```python
from build123d import *

# Parameters (mm, degrees)
SKETCH040_W  = 133
SKETCH040_H  = 133
PAD038_DEPTH = 66.5
PAD039_DEPTH = 5
SKETCH043_W  = 80
SKETCH043_H  = 60
PAD040_DEPTH = 90
PAD046_DEPTH = 5
SKETCH050_W  = 80
SKETCH050_H  = 60
PAD047_DEPTH = 80


with BuildPart() as part:
    # Sketch040 → Pad038 (new body, symmetric)
    with BuildSketch(Plane.XY):
        Rectangle(SKETCH040_W, SKETCH040_H)
    extrude(amount=PAD038_DEPTH, both=True)

    # Sketch041 (on Face6 of Pad038) → Pad039 (join)
    with BuildSketch(Plane.XY.offset(66.5)):
        with BuildLine():
            Line((-88.5, 88.5), (-66.5, 88.5))
            Line((-66.5, 88.5), (-66.5, 67.5))
            ThreePointArc((-67.5, 66.5), (-65.792893, 65.792893), (-66.5, 67.5))
            Line((-88.5, 66.5), (-67.5, 66.5))
            Line((-88.5, 66.5), (-88.5, 88.5))
        make_face()
    extrude(amount=PAD039_DEPTH)

    # Sketch043 (on Face13 of Pad039) → Pad040 (join)
    with BuildSketch(Plane.XY.offset(71.5)):
        with Locations((-77.5, 82.5)):
            Rectangle(SKETCH043_W, SKETCH043_H)
    extrude(amount=PAD040_DEPTH)

    # Sketch049 (on Face13 of Pad040) → Pad046 (join)
    with BuildSketch(Plane.XY.offset(66.5)):
        with BuildLine():
            Line((91, -66.5), (91, -91))
            Line((91, -91), (66.5, -91))
            Line((66.5, -69), (66.5, -91))
            ThreePointArc((69, -66.5), (64.732233, -64.732233), (66.5, -69))
            Line((69, -66.5), (91, -66.5))
        make_face()
    extrude(amount=PAD046_DEPTH)

    # Sketch050 (on Face23 of Pad046) → Pad047 (join)
    with BuildSketch(Plane.XY.offset(71.5)):
        with Locations((78.75, -73.75)):
            Rectangle(SKETCH050_W, SKETCH050_H)
    extrude(amount=PAD047_DEPTH)


solid = part.part
```
The listing builds one solid part. Answer for the finished solid, in the listing's coordinates (mm). A direction names the side the tool comes from. Coordinates: 2 decimals unless noted, no trailing zeros. Write each loop counter-clockwise with the first axis right and the second up, starting at its lowest first coordinate (ties: lowest second). Pieces come first, ordered by that corner, then holes. Notation, with made-up numbers: (75, -25.75) - (116, -25.75) arc R30 ccw to (116, 1.25) - close; hole circle Ø5 at (37, 34). An arc over 180 degrees is marked (long way). One line per item, written item: value.
1) Consider line 1 along Y through (x, z) = (3, -29); line 2 along Z through (x, y) = (41, -83.5). Determine where each line is inside the solid, lowest interval first. Write a range as from..to.
Geometry check:
line 1: y = -66.5..66.5
line 2: z = 71.5..151.5
2) Find section A-A (x = 48). Give the vertices of the cut face in (y, z).
Geometry check:
outline: (-103.75, 71.5) - (-43.75, 71.5) - (-43.75, 151.5) - (-103.75, 151.5) - close; (-66.5, -66.5) - (66.5, -66.5) - (66.5, 66.5) - (-66.5, 66.5) - close
3) Each of these flat-tipped pins is pushed along its axis until it touches: pin 1 Ø4 at (x, z) = (-75, 69) entering from -Y; pin 2 Ø5 at (x, z) = (71, 89) entering from +Y; pin 3 Ø1.5 at (y, z) = (-82, 68) entering from +X; pin 4 Ø12 at (x, z) = (-76, 71) entering from +Y. Where does it stop, or does it pass through?
Geometry check:
pin 1: stops at y = 66.5
pin 2: stops at y = -43.75
pin 3: stops at x = 91
pin 4: stops at y = 112.5
4) A tool of negligible diameter and unlimited length cuts with its end or side. For faces 1 (the flat face through (78, -43.75, 111)), 2 (the flat face through (-1, 66.5, 1)), 3 (the flat face through (-1, -66.5, 1)), 4 (the flat face through (66.5, -1, 1)), from which of +Z, -Z, +X, -X, +Y, -Y can it reach the whole face along a straight path? Write none if from no direction.
Geometry check:
face 1: +Z, +X, -X, +Y
face 2: -Z, +X, -X, +Y
face 3: -Z, +X, -X, -Y
face 4: -Z, +X, +Y, -Y
5) Find section B-B (z = 102.5). Give the vertices of the cut face in (x, y).
Geometry check:
outline: (-117.5, 52.5) - (-37.5, 52.5) - (-37.5, 112.5) - (-117.5, 112.5) - close; (38.75, -103.75) - (118.75, -103.75) - (118.75, -43.75) - (38.75, -43.75) - close
6) Find section C-C (z = -35). Give the vertices of the cut face in (x, y), and give its area (3 significant figures).
Geometry check:
outline: (-66.5, -66.5) - (66.5, -66.5) - (66.5, 66.5) - (-66.5, 66.5) - close
area: 17,700 mm2
